Job drawing, mm, ordinate dimensions from the low corner. One solid piece. A direction names the side the tool comes from. Coordinates: 2 decimals unless noted, no trailing zeros. Write each loop counter-clockwise with the first axis right and the second up, starting at its lowest first coordinate (ties: lowest second). Pieces come first, ordered by that corner, then holes. Notation, with made-up numbers: (43.25, 51.25) - (92.25, 51.25) arc R17 ccw to (92.25, 57.25) - close; hole circle Ø6 at (-4.75, -4.5). An arc over 180 degrees is marked (long way). Put each result on its own line as item: value. Start each with the question number.
1. Drop flat-ended pins along their axis: P1, Ø2, axis at y = 5, z = 2, coming from the +X side; P2, Ø6, axis at x = 11, z = 3.5, coming from the -Y side; P3, Ø3, axis at x = 17, z = 4.5, coming from the +Y side; P4, Ø3, axis at x = 31.5, y = 7, coming from the -Z side. Give the stop position or say it passes through.
2. Saw through at B-B, the plane x = 13. Write the cut outline in (y, z), plus the area to 3 significant figures.
3. Drill centre lines: L1, parallel to Y at x = 17.5, z = 5.75; L2, parallel to X at y = 5, z = 3.75; L3, parallel to Y at x = 15, z = 7. Where is each one in solid material? Low to high. Write a range as from..to.
4. Saw through at C-C, the plane x = 5. Write the cut outline in (y, z).
5. Saw through at A-A, the plane z = 6. Write the cut outline in (x, y), plus the area to 3 significant figures.
6. Which spindle directions (+Z, -Z, +X, -X, +Y, -Y) get a long thin tool onto all of the face, cutting with end or side? Do the marked faces 1 and 2. Say none if no direction does.
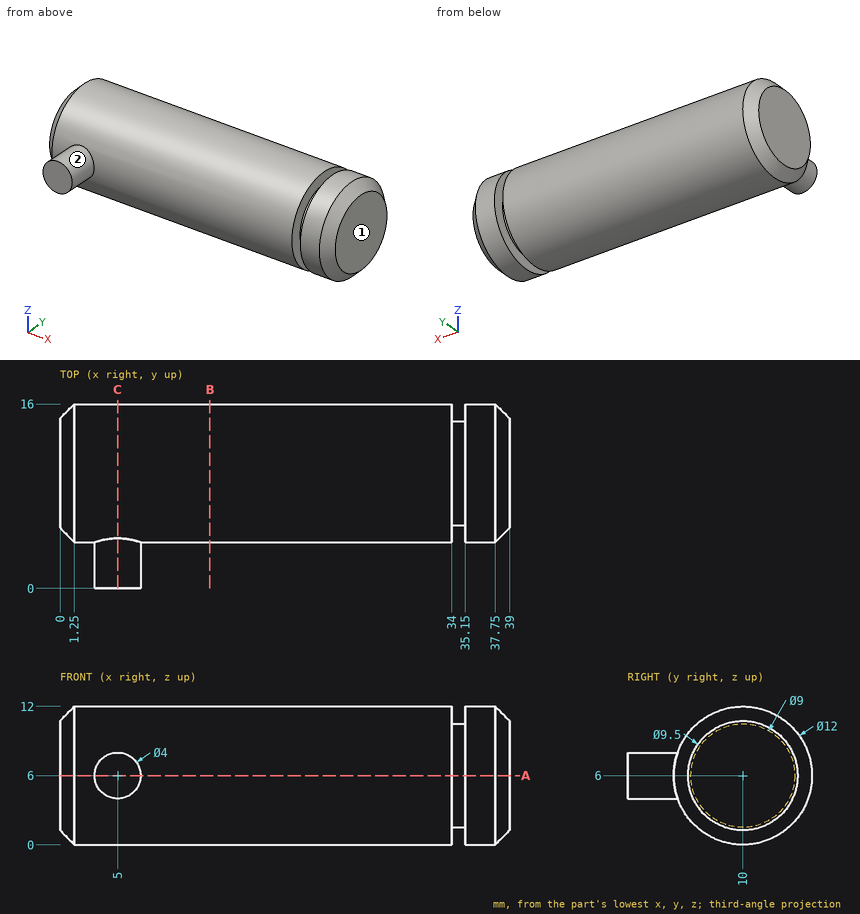
Final values:
1. P1: stops at x = 38.35
1. P2: stops at y = 4
1. P3: stops at y = 16
1. P4: stops at z = 0.19
2. outline: circle Ø12 at (10, 6)
2. area: 113 mm²
3. L1: y = 4.01..15.99
3. L2: x = 0.73..34, 35.15..38.27
3. L3: y = 4.08..15.92
4. outline: (0, 4) - (4.34, 4) arc R6 ccw (long way) to (4.34, 8) - (0, 8) - close
5. outline: (0, 5.25) - (1.25, 4) - (3, 4) - (3, 0) - (7, 0) - (7, 4) - (34, 4) - (34, 5.5) - (35.15, 5.5) - (35.15, 4) - (37.75, 4) - (39, 5.25) - (39, 14.75) - (37.75, 16) - (35.15, 16) - (35.15, 14.5) - (34, 14.5) - (34, 16) - (1.25, 16) - (0, 14.75) - close
5. area: 477 mm²
6. face 1: +Z, -Z, +X, +Y, -Y
6. face 2: -Y
